Build history of the part. All positions in model axes, mm. Face numbers are marked on the shaded views. A direction names the side the tool comes from. Round coordinates to 2 decimals unless told otherwise and drop trailing zeros. Write each loop counter-clockwise with the first axis right and the second up, starting at its lowest first coordinate (ties: lowest second). Pieces come first, ordered by that corner, then holes.
Item 1: Mould opens along X. For the marked faces 1, 2 and 3 say: +X half, -X half, draft (parallel to the pull), parting line (faces both ways), or undercut.
Item 2: Band-saw the part on A-A, the plane z = 0. Write the cut outline in (x, y).
Item 3: 3-axis set-ups, long thin cutter, end or side, ignore diameter. For the marked faces 4, 5 and 6: which of +Z, -Z, +X, -X, +Y, -Y reach the whole face in a straight line?
Item 4: Band-saw the part on B-B, the plane x = 0. Write the cut outline in (y, z), then the cut area to 3 significant figures.
Item 5: Wall check: probe 1 along X at (y, z) = (-1, 0.15); probe 2 along Z at (x, y) = (0.6, -0.75); probe 3 along Z at (x, y) = (-1.4, -0.5). Give the ranges that are in metal, low to high.
Item 6: Band-saw the part on C-C, the plane y = -2.25. Write the cut outline in (x, z).
Item 7: Drop flat-ended pins along their axis: pin 1 Ø0.5 at (y, z) = (-1, 1) entering from +X; pin 2 Ø1 at (x, y) = (-0.5, -2.5) entering from +Z; pin 3 Ø0.9 at (x, y) = (0.5, -0.5) entering from -Z. Give the stop position or say it passes through.
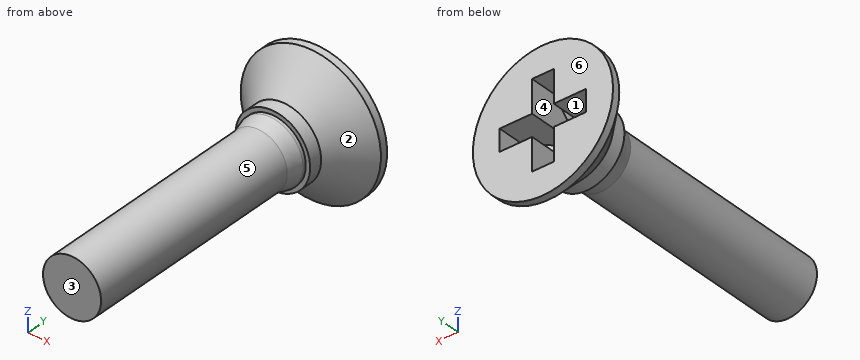
```python
from build123d import *

# Parameters (mm, degrees)
KREUZSCHLITZ1_H_DEPTH      = 0.363
KREUZSCHLITZ1_H_DEPTH_BACK = 0.363
KREUZSCHLITZ2_H_DEPTH      = 0.363
KREUZSCHLITZ2_H_DEPTH_BACK = 0.363


with BuildPart() as part:
    # Skizze1 → Basis-Rotation (revolve)
    with BuildSketch(Plane.XY, mode=Mode.PRIVATE) as basis_rotation_sk:
        Polygon((0, 0), (2.35, 0), (2.35, -0.254), (1.25, -1.354), (1.25, -1.804), (1.104, -1.804), (1.104, -1.914833395), (0.974, -2.4), (0.974, -10), (0, -10), align=None)
    revolve(basis_rotation_sk.sketch.rotate(Axis((0, 0, 0), (0, -1, 0)), 180), axis=Axis((0, 0, 0), (0, -1, 0)))

    # Skizze2 → Kreuzschlitz1 H (cut, two sides: drawn at the far end of the back side and taken through both)
    with BuildSketch(Plane.XY.offset(-KREUZSCHLITZ1_H_DEPTH_BACK)):
        Polygon((-0.55, -1.8), (0.55, -1.8), (1.45, -0.9), (1.45, 0), (-1.45, 0), (-1.45, -0.9), align=None)
    extrude(amount=KREUZSCHLITZ1_H_DEPTH + KREUZSCHLITZ1_H_DEPTH_BACK, mode=Mode.SUBTRACT)

    # Skizze3 → Kreuzschlitz2 H (cut, two sides: drawn at the far end of the back side and taken through both)
    with BuildSketch(Plane(origin=(0, 0, 0), x_dir=(0, 0, -1), z_dir=(1, 0, 0)).offset(-KREUZSCHLITZ2_H_DEPTH_BACK)):
        Polygon((-0.55, -1.8), (0.55, -1.8), (1.45, -0.9), (1.45, 0), (-1.45, 0), (-1.45, -0.9), align=None)
    extrude(amount=KREUZSCHLITZ2_H_DEPTH + KREUZSCHLITZ2_H_DEPTH_BACK, mode=Mode.SUBTRACT)


solid = part.part
```
Results:
1. face 1: undercut
1. face 2: parting line
1. face 3: draft
2. outline: (-2.35, -0.25) - (-1.25, -1.35) - (-1.25, -1.8) - (-1.1, -1.8) - (-1.1, -1.91) - (-0.97, -2.4) - (-0.97, -10) - (0.97, -10) - (0.97, -2.4) - (1.1, -1.91) - (1.1, -1.8) - (1.25, -1.8) - (1.25, -1.35) - (2.35, -0.25) - (2.35, 0) - (1.45, 0) - (1.45, -0.9) - (0.55, -1.8) - (-0.55, -1.8) - (-1.45, -0.9) - (-1.45, 0) - (-2.35, 0) - close
3. face 4: +Y
3. face 5: -Y
3. face 6: +Z, -Z, +X, -X, +Y
4. outline: (-10, -0.97) - (-2.4, -0.97) - (-1.91, -1.1) - (-1.8, -1.1) - (-1.8, -1.25) - (-1.35, -1.25) - (-0.25, -2.35) - (0, -2.35) - (0, -1.45) - (-0.9, -1.45) - (-1.8, -0.55) - (-1.8, 0.55) - (-0.9, 1.45) - (0, 1.45) - (0, 2.35) - (-0.25, 2.35) - (-1.35, 1.25) - (-1.8, 1.25) - (-1.8, 1.1) - (-1.91, 1.1) - (-2.4, 0.97) - (-10, 0.97) - close
4. area: 17.9 mm2
5. probe 1: x = -1.6 to -1.35, 1.35 to 1.6
5. probe 2: z = -1.75 to -0.36, 0.36 to 1.75
5. probe 3: z = -1.57 to -0.36, 0.36 to 1.57
6. outline: circle Ø2.03 at (0, 0)
7. pin 1: stops at x = 1.6
7. pin 2: stops at z = 1.04
7. pin 3: stops at z = -2.35
